Could you check a few things on this drawing? It's one solid part, dimensions in mm from its lowest x, y, z. Coordinates: 2 decimals unless noted, no trailing zeros. Write each loop counter-clockwise with the first axis right and the second up, starting at its lowest first coordinate (ties: lowest second). Pieces come first, ordered by that corner, then holes. Notation, with made-up numbers: (79.5, 31.5) - (102.5, 31.5) arc R26 cw to (102.5, 66.5) - close; hole circle Ø5 at (52, 11). An arc over 180 degrees is marked (long way). Answer as a JSON object with one key per item and string values. Group by question number.
1) Will this pin go through, and if not, where does the flat tip stop? pin 1 Ø9 at (x, y) = (15, 15) entering from +Z.
2) If we section it at A-A (y = 155): Write out the boundary of the cut face in (x, z), plus the area to 3 significant figures.
3) Please list where these lines run through material, in increasing order: line 1 along X through (y, z) = (15, 2); line 2 along X through (y, z) = (21, 3.75).
4) If we section it at C-C (z = 1.5): Write out the boundary of the cut face in (x, y), plus the area to 3 significant figures.
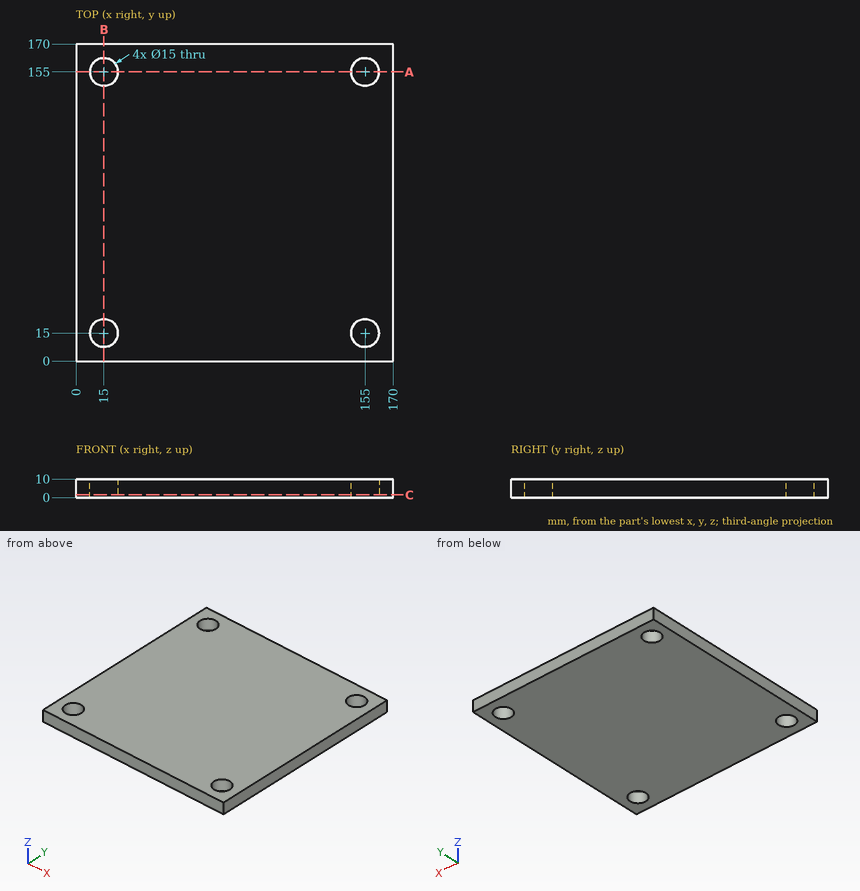
Here are the results:
{
 "1": {"pin 1": "passes through"},
 "2": {"outline": "(0, 0) - (7.5, 0) - (7.5, 10) - (0, 10) - close; (22.5, 0) - (147.5, 0) - (147.5, 10) - (22.5, 10) - close; (162.5, 0) - (170, 0) - (170, 10) - (162.5, 10) - close", "area": "1,400 mm²"},
 "3": {"line 1": "x = 0 to 7.5, 22.5 to 147.5, 162.5 to 170", "line 2": "x = 0 to 10.5, 19.5 to 150.5, 159.5 to 170"},
 "4": {"outline": "(0, 0) - (170, 0) - (170, 170) - (0, 170) - close; hole circle Ø15 at (15, 15); hole circle Ø15 at (15, 155); hole circle Ø15 at (155, 15); hole circle Ø15 at (155, 155)", "area": "28,200 mm²"}
}
